from build123d import *

# Parameters (mm, degrees)
F1_DEPTH = 25.4


with BuildPart() as f1:
    # F0 (on Front) → F1 (new body)
    with BuildSketch(Plane.XZ):
        with BuildLine():
            ThreePointArc((-39.140027, 35.391811), (-36.560582, 37.734512), (-33.085216, 37.986729))
            Line((-33.085216, 37.986729), (-33.085216, 12.902514))
            ThreePointArc((-33.085216, 12.902514), (-31.90952, 5.966876), (-28.183702, 0))
            Line((-28.183702, 0), (-14.055812, -15.064946))
            ThreePointArc((-14.055812, -15.064946), (-7.648839, -19.397211), (0, -20.543108))
            Line((0, -20.543108), (6.70354, -20.543108))
            ThreePointArc((6.70354, -20.543108), (11.677188, -18.411115), (15.929919, -15.064946))
            Line((15.929919, -15.064946), (30.634461, 0))
            ThreePointArc((30.634461, 0), (33.004035, 7.146345), (33.806026, 14.632461))
            Line((33.806026, 14.632461), (33.806026, 37.986729))
            ThreePointArc((33.806026, 37.986729), (36.68927, 39.789823), (39.572515, 37.986729))
            Line((39.572515, 37.986729), (50.240513, 16.074082))
            ThreePointArc((50.240513, 16.074082), (57.20934, 16.529722), (62.061809, 21.552242))
            Line((62.061809, 21.552242), (67.539975, 34.526836))
            ThreePointArc((67.539975, 34.526836), (66.722582, 39.70047), (63.791759, 44.04154))
            Line((63.791759, 44.04154), (52.835435, 54.421216))
            Line((52.835435, 54.421216), (25.156297, 54.421216))
            Line((25.156297, 54.421216), (22.849701, 54.421216))
            Line((22.849701, 54.421216), (5.261919, 54.421216))
            Line((5.261919, 54.421216), (-50.096352, 54.421216))
            Line((-50.096352, 54.421216), (-61.340999, 42.023271))
            ThreePointArc((-61.340999, 42.023271), (-63.167493, 38.335649), (-62.782623, 34.238514))
            Line((-62.782623, 34.238514), (-59.899379, 21.552242))
            ThreePointArc((-59.899379, 21.552242), (-56.794074, 16.484717), (-51.249649, 14.344135))
            Line((-51.249649, 14.344135), (-45.771487, 23.282189))
            Line((-45.771487, 23.282189), (-39.140027, 35.391811))
        make_face()
        with BuildLine():
            Line((-15.785757, 7.712676), (-9.452744, 7.712676))
            Line((-9.452744, 7.712676), (17.083218, 7.712676))
            ThreePointArc((17.083218, 7.712676), (12.289972, 7.202582), (7.711429, 5.695148))
            Line((7.711429, 5.695148), (7.711429, -7.280189))
            ThreePointArc((7.711429, -7.280189), (4.918177, -11.449271), (0, -10.451756))
            ThreePointArc((0, -10.451756), (-5.866974, -12.265498), (-9.452744, -7.280189))
            Line((-9.452744, -7.280189), (-9.452744, 6.684112))
            ThreePointArc((-9.452744, 6.684112), (-12.577759, 7.453861), (-15.785757, 7.712676))
        make_face(mode=Mode.SUBTRACT)
        with BuildLine():
            Line((-9.442623, 24.723811), (-5.982729, 25.300462))
            Line((-5.982729, 25.300462), (9.010135, 25.300462))
            ThreePointArc((9.010135, 25.300462), (5.448393, 18.275855), (-1.534213, 14.632461))
            ThreePointArc((-1.534213, 14.632461), (-7.400178, 18.179924), (-9.442623, 24.723811))
        make_face(mode=Mode.SUBTRACT)
        with BuildLine():
            Line((-19.245649, 32.220244), (-19.245649, 43.753218))
            ThreePointArc((-19.245649, 43.753218), (-14.344136, 45.695412), (-9.442623, 43.753218))
            Line((-9.442623, 43.753218), (-9.452744, 32.220244))
            ThreePointArc((-9.452744, 32.220244), (-10.616261, 29.266754), (-13.479163, 27.895378))
            ThreePointArc((-13.479163, 27.895378), (-17.443622, 28.61619), (-19.245649, 32.220244))
        make_face(mode=Mode.SUBTRACT)
        with BuildLine():
            Line((12.181703, 31.355269), (12.181703, 45.194838))
            ThreePointArc((12.181703, 45.194838), (16.218243, 49.231378), (20.254783, 45.194838))
            Line((20.254783, 45.194838), (20.254783, 31.355269))
            ThreePointArc((20.254783, 31.355269), (16.218243, 27.318729), (12.181703, 31.355269))
        make_face(mode=Mode.SUBTRACT)
    extrude(amount=F1_DEPTH)


solid = f1.part
The listing builds one solid part. Answer for the finished solid, in the listing's coordinates (mm). A direction names the side the tool comes from. Coordinates: 2 decimals unless noted, no trailing zeros. Order: outer loops, then holes, each group sorted by start corner. A loop starts at its lowest first (then second) coordinate and runs counter-clockwise, first axis right, second up.
Q1. A cutting plane is placed at D-D, the plane x = 46. Write down the section's boundary in (y, z), and give its area (3 significant figures).
Q2. Given P1, Ø2, axis at y = -2.5, z = 40, coming from the -X side; P2, Ø14.5, axis at y = -13.5, z = -0.5, coming from the -X side; P3, Ø6, axis at y = -8.5, z = 39, coming from the +X side, each flat-ended and moving along its own axis, determine where each tip first touches the part or whether it passes through.
Q3. A cutting plane is placed at A-A, the plane z = 47.5. Write down the section's boundary in (x, y).
Q4. A cutting plane is placed at B-B, the plane x = 19. Write down the section's boundary in (y, z).
Q5. For a pull along Z with two mould halves and no side action, classify faces 1 (the face through (16.13, -12.52, 49.23)), 2 (the face through (5.53, -12.52, 18.36)), 3 (the face through (-42.502, -12.522, 29.252)), 4 (the face through (2, -13, 54.421)) as pulls with the +Z half, pulls with the -Z half, needs draft (parallel to the pull), parting line crosses it, or undercut.
Q6. Which of the six approach directions +Z, -Z, +X, -X, +Y, -Y give full straight-line access (tool end or side, diameter ignored) to faces 5 (the face through (-55.64, -12.52, 48.31)), 6 (the face through (-7.339, -12.522, 18.103)), 7 (the face through (-48.55, -12.52, 18.75))?
Q7. Consider line 1 (X direction, y = -16, z = 43.5); line 2 (Z direction, x = -13, y = -14.5); line 3 (Z direction, x = -8.5, y = -14.75). Determine where each line is inside the solid, lowest interval first.
Q8. A cutting plane is placed at C-C, the plane y = -5. State how many separate pieces and enclosed holes the cut face has, and give its area (3 significant figures).
Answers follow:
1. outline: (-25.4, 24.78) - (0, 24.78) - (0, 54.42) - (-25.4, 54.42) - close
1. area: 753 mm2
2. P1: stops at x = -63.01
2. P2: stops at x = -32.19
2. P3: stops at x = 67.54
3. outline: (-56.37, -25.4) - (12.9, -25.4) - (12.9, 0) - (-56.37, 0) - close; (19.53, -25.4) - (60.14, -25.4) - (60.14, 0) - (19.53, 0) - close
4. outline: (-25.4, -11.92) - (0, -11.92) - (0, 28.43) - (-25.4, 28.43) - close; (-25.4, 48.12) - (0, 48.12) - (0, 54.42) - (-25.4, 54.42) - close
5. face 1: undercut
5. face 2: undercut
5. face 3: pulls with the -Z half
5. face 4: pulls with the +Z half
6. face 5: +Z, -X, +Y, -Y
6. face 6: +Y, -Y
6. face 7: -Z, +Y, -Y
7. line 1: x = -60 to -19.25, -9.44 to 12.18, 20.25 to 64.33
7. line 2: z = -16.1 to 7.52, 7.71 to 27.96, 45.57 to 54.42
7. line 3: z = -19.04 to -10.3, 7.71 to 19.95, 24.88 to 54.42
8. separate pieces: 1
8. enclosed holes: 4
8. area: 5,240 mm2
